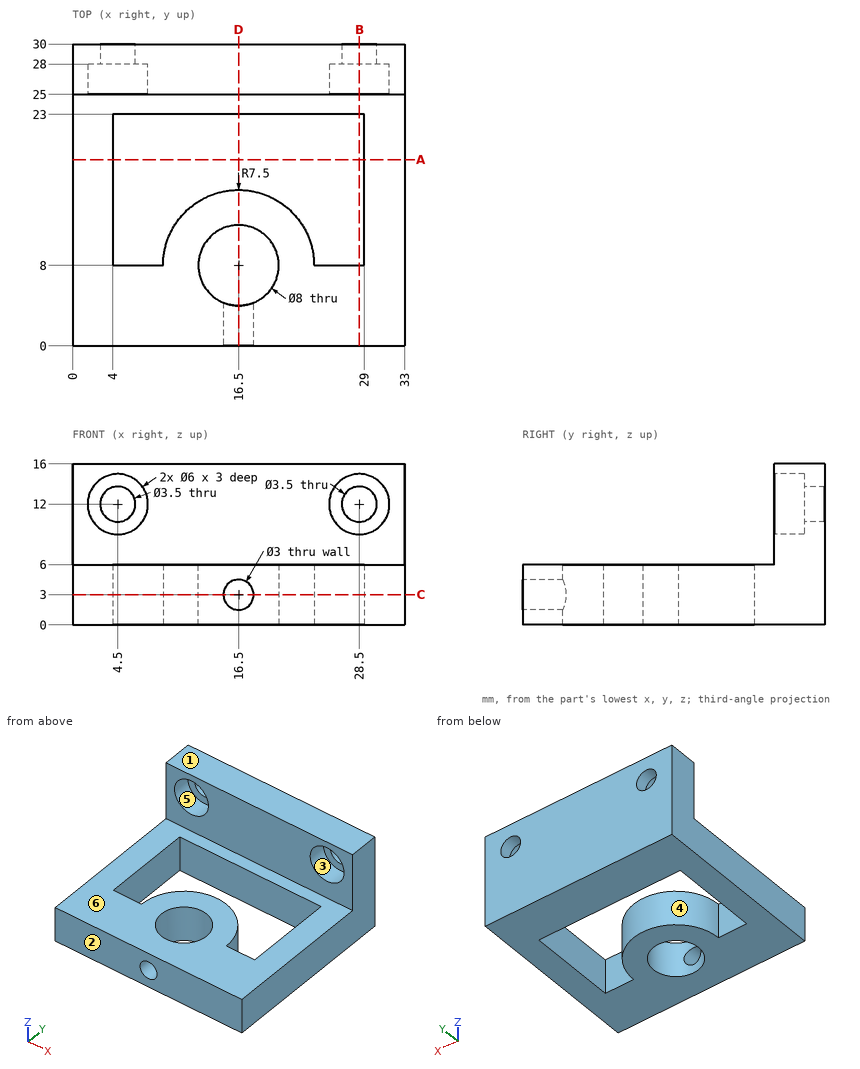
For this review, use the dimensioned drawing (mm, ordinates from the lowest corner) and the shaded views. A direction names the side the tool comes from. Coordinates: 2 decimals unless noted, no trailing zeros. Loops run counter-clockwise (first coordinate to the right, second up) from the corner with the lowest first, then second, coordinate; pieces in that order, holes last. Notation, with made-up numbers: (15.25, 4.25) -> (68.25, 4.25) arc R15 ccw to (68.25, 13.25) -> close; hole circle Ø8 at (61, 13). An arc over 180 degrees is marked (long way). Use a Markdown table: item, result. Add a question column.
1. Clearance check with flat-ended pins moving along their axes: pin 1 Ø3 at (x, z) = (21, 9) entering from -Y; pin 2 Ø3 at (y, z) = (20.5, 8) entering from +X; pin 3 Ø8 at (x, y) = (21.5, 16.5) entering from +Z. State where each tip first meets the part, or that it passes through.
2. Add section B-B on x = 28.5. Write out the cut boundary in (y, z).
3. Add section D-D on x = 16.5. Write out the cut boundary in (y, z).
4. To check wall thickness, follow line 1 (Z direction, x = 28.5, y = 26.45); line 2 (Z direction, x = 16.5, y = 1.7). State the ranges of each line that lie inside material, in increasing order.
5. Add section A-A on y = 18.5. Write out the cut boundary in (x, z).
6. Add section C-C on z = 3. Write out the cut boundary in (x, y), plus the area to 3 significant figures.
7. Draft analysis for pull direction Z (two halves, no side actions). For the marked faces 1, 2 and 3, state which applies: pulls with the +Z half, pulls with the -Z half, needs draft (parallel to the pull), parting line crosses it, or undercut.
8. Machinability: for the marked faces 4, 5 and 6, which of the approach directions +Z, -Z, +X, -X, +Y, -Y give a long, thin tool a straight path to every point of the face, cutting with its end or side? Answer none if there is none.
Returned:
| question | item | result |
|---|---|---|
| 1 | pin 1 | stops at y = 25 |
| 1 | pin 2 | passes through |
| 1 | pin 3 | stops at z = 6 |
| 2 | outline | (0, 0) -> (8, 0) -> (8, 6) -> (0, 6) -> close; (23, 0) -> (30, 0) -> (30, 10.25) -> (28, 10.25) -> (28, 9) -> (25, 9) -> (25, 6) -> (23, 6) -> close; (25, 15) -> (28, 15) -> (28, 13.75) -> (30, 13.75) -> (30, 16) -> (25, 16) -> close |
| 3 | outline | (0, 0) -> (4, 0) -> (4, 1.5) -> (0, 1.5) -> close; (0, 4.5) -> (4, 4.5) -> (4, 6) -> (0, 6) -> close; (12, 0) -> (15.5, 0) -> (15.5, 6) -> (12, 6) -> close; (23, 0) -> (30, 0) -> (30, 16) -> (25, 16) -> (25, 6) -> (23, 6) -> close |
| 4 | line 1 | z = 0 to 9, 15 to 16 |
| 4 | line 2 | z = 0 to 1.5, 4.5 to 6 |
| 5 | outline | (0, 0) -> (4, 0) -> (4, 6) -> (0, 6) -> close; (29, 0) -> (33, 0) -> (33, 6) -> (29, 6) -> close |
| 6 | outline | (0, 0) -> (15, 0) -> (15, 4.29) arc R4 cw (long way) to (18, 4.29) -> (18, 0) -> (33, 0) -> (33, 30) -> (0, 30) -> close; hole (4, 8) -> (9, 8) arc R7.5 cw to (24, 8) -> (29, 8) -> (29, 23) -> (4, 23) -> close |
| 6 | area | 641 mm² |
| 7 | face 1 | pulls with the +Z half |
| 7 | face 2 | needs draft |
| 7 | face 3 | undercut |
| 8 | face 4 | +Z, -Z |
| 8 | face 5 | -Y |
| 8 | face 6 | +Z, +X, -X, -Y |
